```python
from build123d import *

# Parameters (mm, degrees)
SKETCH009_R     = 7.15
PAD009_DEPTH    = 7
PAD010_DEPTH    = 12
SKETCH011_W     = 4.95
SKETCH011_H     = 3
POCKET_DEPTH    = 19.001
CHAMFER_SIZE    = 1.5
CHAMFER001_SIZE = 1


with BuildPart() as part:
    # Sketch009 → Pad009 (new body)
    with BuildSketch(Plane.XY):
        with Locations((84.022852, 0)):
            Circle(SKETCH009_R)
    extrude(amount=PAD009_DEPTH)

    # Sketch010 (on Face2 of Pad009) → Pad010 (join)
    with BuildSketch(Plane(origin=(0, 0, 0), x_dir=(1, 0, 0), z_dir=(0, 0, -1))):
        with BuildLine():
            ThreePointArc((90.872852, -8.349701), (84.022852, 10.8), (77.172852, -8.349701))
            Line((79.487898, -5.527811), (77.172852, -8.349701))
            ThreePointArc((79.487898, -5.527811), (84.022852, -7.15), (88.557806, -5.527811))
            Line((88.557806, -5.527811), (90.872852, -8.349701))
        make_face()
    extrude(amount=PAD010_DEPTH)

    # Sketch011 (on Face8 of Pad010) → Pocket (cut, through all)
    with BuildSketch(Plane(origin=(0, 0, -12), x_dir=(1, 0, 0), z_dir=(0, 0, -1))):
        with Locations((84.022852, 0)):
            Rectangle(SKETCH011_W, SKETCH011_H)
    extrude(amount=-POCKET_DEPTH, mode=Mode.SUBTRACT)

    # Chamfer
    chamfer_edges = [part.edges().sort_by_distance(p)[0] for p in [
        (84.022852, -10.8, -12),
    ]]
    chamfer(chamfer_edges, length=CHAMFER_SIZE)

    # Chamfer001
    chamfer001_edges = [part.edges().sort_by_distance(p)[0] for p in [
        (84.022852, -10.8, 0),
    ]]
    chamfer(chamfer001_edges, length=CHAMFER001_SIZE)


solid = part.part
```
For this review, take the finished solid that the model builds, in its own axes (mm). A direction names the side the tool comes from. Coordinates: 2 decimals unless noted, no trailing zeros. Write each loop counter-clockwise with the first axis right and the second up, starting at its lowest first coordinate (ties: lowest second). Pieces come first, ordered by that corner, then holes. Notation, with made-up numbers: (12.25, 19.25) - (35.25, 19.25) arc R24 cw to (35.25, 29.25) - close; hole circle Ø11 at (8, -12.75). An arc over 180 degrees is marked (long way). Answer in a Markdown table with one row per item. Add a question column.
Q1. For P1, Ø10, axis at x = 80, z = -0.5, coming from the -Y side; P2, Ø1.5, axis at x = 78, z = 1.5, coming from the -Y side; P3, Ø1.5, axis at x = 80, z = 0, coming from the -Y side; P4, Ø1.5, axis at x = 90.5, z = 1, coming from the +Y side, all flat-tipped, find the tip position at first contact; note any pin that passes through.
Q2. Tool access review of faces 4 (the conical face through (84.351, -9.534, -11.761)), 5 (the flat face through (78.347, 6.919, -5.916)), 6 (the flat face through (86.498, 0, -3)): name each direction out of +Z, -Z, +X, -X, +Y, -Y from which nothing blocks a thin tool from reaching the whole face with its end or side.
Q3. Draft analysis for pull direction X (two halves, no side actions). For faces 1 (the flat face through (84, -3, -12)), 2 (the flat face through (84, 1.5, -3)), 3 (the conical face through (84.365, -9.954, -0.16)), state which applies: +X half, -X half, draft (parallel to the pull), parting line (faces both ways), or undercut.
Q4. We need section B-B, the plane y = 0. State the section outline as (x, z) points.
Q5. We need section C-C, the plane z = 0.5. State the section outline as (x, y) points, and give its area (3 significant figures).
Q6. For probe 1 along Y at (x, z) = (84.25, -1.25); probe 2 along Z at (x, y) = (84.25, -8.25); probe 3 along X at (y, z) = (7.75, -1.25), list the stretches that pass through material, from the lowest coordinate up.
Q7. We need section A-A, the plane z = -5.25. State the section outline as (x, y) points, and give its area (3 significant figures).
Answer list:
| question | item | result |
|---|---|---|
| 1 | P1 | stops at y = -10.8 |
| 1 | P2 | stops at y = -4.83 |
| 1 | P3 | stops at y = -9.81 |
| 1 | P4 | stops at y = 4.28 |
| 2 | face 4 | -Z |
| 2 | face 5 | +Z, -Z, +Y |
| 2 | face 6 | +Z, -Z |
| 3 | face 1 | draft |
| 3 | face 2 | undercut |
| 3 | face 3 | parting line |
| 4 | outline | (73.22, -10.5) - (74.72, -12) - (81.55, -12) - (81.55, 7) - (76.87, 7) - (76.87, 0) - (74.22, 0) - (73.22, -1) - close; (86.5, -12) - (93.32, -12) - (94.82, -10.5) - (94.82, -1) - (93.82, 0) - (91.17, 0) - (91.17, 7) - (86.5, 7) - close |
| 5 | outline | circle Ø14.3 at (84.02, 0); hole (81.55, -1.5) - (86.5, -1.5) - (86.5, 1.5) - (81.55, 1.5) - close |
| 5 | area | 146 mm2 |
| 6 | probe 1 | y = -10.8 to -1.5, 1.5 to 7.15 |
| 6 | probe 2 | z = -12 to 0 |
| 6 | probe 3 | x = 76.5 to 77.66, 90.38 to 91.54 |
| 7 | outline | (77.17, 8.35) arc R10.8 ccw (long way) to (90.87, 8.35) - (88.56, 5.53) arc R7.15 ccw to (79.49, 5.53) - close; hole (81.55, -1.5) - (86.5, -1.5) - (86.5, 1.5) - (81.55, 1.5) - close |
| 7 | area | 307 mm2 |
